Check sheet for the modelled part. Datum: model origin and axes. Units: mm. A direction names the side the tool comes from. Give positions to 0.01 mm unless a question says otherwise; leave off trailing zeros. Write each loop counter-clockwise with the first axis right and the second up, starting at its lowest first coordinate (ties: lowest second). Pieces come first, ordered by that corner, then holes. Notation, with made-up numbers: (-23, 22.25) -> (-7, 22.25) arc R27 ccw to (-7, 50.25) -> close; hole circle Ø9 at (17, 52). An arc over 180 degrees is marked (long way). Return JSON: item names as keys, results as strings.
from build123d import *

# Parameters (mm, degrees)
F0_W      = 690
F0_H      = 350
F0_H_2    = 200
F1_DEPTH  = 80
F2_R      = 25
F2_R_2    = 75
F3_DEPTH  = 100
F4_R      = 75
F5_DEPTH  = 150
F6_R      = 82.5
F6_R_2    = 9
F6_R_3    = 25
F7_DEPTH  = 25
F8_R      = 50
F8_R_2    = 25
F9_DEPTH  = 5
F10_R     = 75
F11_DEPTH = 25
F12_R     = 37.5
F13_DEPTH = 100
F14_R     = 92.5
F14_R_2   = 9
F14_R_3   = 37.5
F15_DEPTH = 25
F16_R     = 60
F16_R_2   = 37.5
F17_DEPTH = 5
F18_W     = 930
F18_H     = 1000
F19_DEPTH = 100
F20_R     = 7
F21_DEPTH = 50


with BuildPart() as f1:
    # F0 (on Front) → F1 (new body)
    with BuildSketch(Plane.XZ):
        Polygon((345, -965), (465, -965), (465, 965), (-465, 965), (-465, -965), (-345, -965), (-345, -765), (345, -765), align=None)
        with Locations((0, -470)):
            Rectangle(F0_W, F0_H, mode=Mode.SUBTRACT)
        with Locations((0, -75)):
            Rectangle(F0_W, F0_H_2, mode=Mode.SUBTRACT)
    extrude(amount=F1_DEPTH)

    # F2 (on face) → F3 (cut)
    with BuildSketch(Plane.XZ.offset(80)):
        with Locations((-300, 125)):
            Circle(F2_R)
        with Locations((0, 425)):
            Circle(F2_R_2)
        with Locations((-300, 725)):
            Circle(F2_R)
        with Locations((300, 125)):
            Circle(F2_R)
        with Locations((300, 725)):
            Circle(F2_R)
    extrude(amount=-F3_DEPTH, mode=Mode.SUBTRACT)

    # F4 (on face) → F5 (join)
    with BuildSketch(Plane.XZ.offset(80)):
        with Locations((-370, 415)):
            Circle(F4_R)
        with Locations((370, 415)):
            Circle(F4_R)
    extrude(amount=F5_DEPTH)

    # F6 (on face) → F7 (join)
    with BuildSketch(Plane.XZ.offset(80)):
        with Locations((-300, 725)):
            Circle(F6_R)
        with Locations((-300, 662.5)):
            Circle(F6_R_2, mode=Mode.SUBTRACT)
        with Locations((-362.5, 725)):
            Circle(F6_R_2, mode=Mode.SUBTRACT)
        with Locations((-300, 725)):
            Circle(F6_R_3, mode=Mode.SUBTRACT)
        with Locations((-300, 787.5)):
            Circle(F6_R_2, mode=Mode.SUBTRACT)
        with Locations((-237.5, 725)):
            Circle(F6_R_2, mode=Mode.SUBTRACT)
        with Locations((-300, 125)):
            Circle(F6_R)
        with Locations((-300, 62.5)):
            Circle(F6_R_2, mode=Mode.SUBTRACT)
        with Locations((-362.5, 125)):
            Circle(F6_R_2, mode=Mode.SUBTRACT)
        with Locations((-300, 125)):
            Circle(F6_R_3, mode=Mode.SUBTRACT)
        with Locations((-237.5, 125)):
            Circle(F6_R_2, mode=Mode.SUBTRACT)
        with Locations((-300, 187.5)):
            Circle(F6_R_2, mode=Mode.SUBTRACT)
        with Locations((300, 725)):
            Circle(F6_R)
        with Locations((300, 662.5)):
            Circle(F6_R_2, mode=Mode.SUBTRACT)
        with Locations((237.5, 725)):
            Circle(F6_R_2, mode=Mode.SUBTRACT)
        with Locations((300, 725)):
            Circle(F6_R_3, mode=Mode.SUBTRACT)
        with Locations((362.5, 725)):
            Circle(F6_R_2, mode=Mode.SUBTRACT)
        with Locations((300, 787.5)):
            Circle(F6_R_2, mode=Mode.SUBTRACT)
        with Locations((300, 125)):
            Circle(F6_R)
        with Locations((237.5, 125)):
            Circle(F6_R_2, mode=Mode.SUBTRACT)
        with Locations((300, 62.5)):
            Circle(F6_R_2, mode=Mode.SUBTRACT)
        with Locations((300, 125)):
            Circle(F6_R_3, mode=Mode.SUBTRACT)
        with Locations((362.5, 125)):
            Circle(F6_R_2, mode=Mode.SUBTRACT)
        with Locations((300, 187.5)):
            Circle(F6_R_2, mode=Mode.SUBTRACT)
    extrude(amount=F7_DEPTH)

    # F8 (on face) → F9 (join)
    with BuildSketch(Plane.XZ.offset(105)):
        with Locations((-300, 725)):
            Circle(F8_R)
        with Locations((-300, 725)):
            Circle(F8_R_2, mode=Mode.SUBTRACT)
        with Locations((-300, 125)):
            Circle(F8_R)
        with Locations((-300, 125)):
            Circle(F8_R_2, mode=Mode.SUBTRACT)
        with Locations((300, 725)):
            Circle(F8_R)
        with Locations((300, 725)):
            Circle(F8_R_2, mode=Mode.SUBTRACT)
        with Locations((300, 125)):
            Circle(F8_R)
        with Locations((300, 125)):
            Circle(F8_R_2, mode=Mode.SUBTRACT)
    extrude(amount=F9_DEPTH)

    # F10 (on face) → F11 (join)
    with BuildSketch(Plane.XZ.offset(80)):
        with Locations((0, 425)):
            Circle(F10_R)
    extrude(amount=-F11_DEPTH)

    # F12 (on face) → F13 (cut)
    with BuildSketch(Plane.XZ.offset(80)):
        with Locations((0, 850)):
            Circle(F12_R)
    extrude(amount=-F13_DEPTH, mode=Mode.SUBTRACT)

    # F14 (on face) → F15 (join)
    with BuildSketch(Plane.XZ.offset(80)):
        with Locations((0, 850)):
            Circle(F14_R)
        with Locations((-72.5, 850)):
            Circle(F14_R_2, mode=Mode.SUBTRACT)
        with Locations((0, 777.5)):
            Circle(F14_R_2, mode=Mode.SUBTRACT)
        with Locations((0, 850)):
            Circle(F14_R_3, mode=Mode.SUBTRACT)
        with Locations((0, 922.5)):
            Circle(F14_R_2, mode=Mode.SUBTRACT)
        with Locations((72.5, 850)):
            Circle(F14_R_2, mode=Mode.SUBTRACT)
    extrude(amount=F15_DEPTH)

    # F16 (on face) → F17 (join)
    with BuildSketch(Plane.XZ.offset(105)):
        with Locations((0, 850)):
            Circle(F16_R)
        with Locations((0, 850)):
            Circle(F16_R_2, mode=Mode.SUBTRACT)
    extrude(amount=F17_DEPTH)

    # F18 (on face) → F19 (cut)
    with BuildSketch(Plane.XZ.offset(80)):
        with Locations((0, -465)):
            Rectangle(F18_W, F18_H)
    extrude(amount=-F19_DEPTH, mode=Mode.SUBTRACT)

    # F20 (on face) → F21 (cut)
    with BuildSketch(Plane(origin=(0, 0, 35), x_dir=(1, 0, 0), z_dir=(0, 0, -1))):
        with Locations((-400, 40)):
            Circle(F20_R)
        with Locations((400, 40)):
            Circle(F20_R)
    extrude(amount=-F21_DEPTH, mode=Mode.SUBTRACT)


solid = f1.part
(1) Release check for a two-part mould opening along Z. For faces 6 (the flat face through (-264, -105, 689)), 7 (the cylindrical face through (-12.042, -92.325, 941.713)), 8 (the flat face through (60.4, -105, 851.3)) record: pulls with the +Z half, pulls with the -Z half, needs draft (parallel to the pull), parting line crosses it, or undercut.
Reply:
{"face 6": "undercut", "face 7": "parting line crosses it", "face 8": "needs draft"}
(2) Cross-section at A-A on y = -93.5. State how many separate pieces and enclosed holes the cut face has, then the cut area to 3 significant figures.
Reply:
{"separate pieces": "7", "enclosed holes": "25", "area": "130,000 mm^2"}
(3) Set-up check for faces 1 (the cylindrical face through (-9.764, -27.885, 499.362)), 2 (the flat face through (7, -39, 965)), 3 (the flat face through (310.4, -110, 147.9)), 4 (the cylindrical face through (-349.95, -107.46, 127.2)), 5 (the flat face through (277.1, -110, 714.6)): record each of +Z, -Z, +X, -X, +Y, -Y from which the full face is reachable in a straight line by a thin tool's end or side.
Reply:
{"face 1": "+Y", "face 2": "+Z, +X, -X, +Y, -Y", "face 3": "-Z, +X, -X, -Y", "face 4": "-Y", "face 5": "+Z, +X, -X, -Y"}
(4) Cross-section at B-B on z = 626.5. Enter the section's corners in (x, y).
Reply:
{"outline": "(-465, -80) -> (465, -80) -> (465, 0) -> (-465, 0) -> close"}
(5) Thickness scan on L1, parallel to Z at x = -303.5, y = -26.5; L2, parallel to Z at x = 0, y = -29; L3, parallel to X at y = -115, z = 410.5. Record the ranges inside material, lowest first.
Reply:
{"L1": "35 to 100.25, 149.75 to 700.25, 749.75 to 965", "L2": "35 to 350, 500 to 812.5, 887.5 to 965", "L3": "-444.86 to -295.14, 295.14 to 444.86"}
(6) Depth check by flat-ended pin: pin 1 Ø2 at (x, z) = (222, 762.5) entering from -Y; pin 2 Ø2 at (x, y) = (312.5, -109.5) entering from +Z; pin 3 Ø20.5 at (x, z) = (-300, 787.5) entering from -Y. Enter the tip coordinate at first touch or a pass-through.
Reply:
{"pin 1": "y = -80", "pin 2": "z = 773.66", "pin 3": "y = -105"}
